Source: CAD feature listing. Evaluate the final solid. Frame: model axes, mm. Give positions to 0.01 mm unless a question says otherwise; leave off trailing zeros. Write each loop counter-clockwise with the first axis right and the second up, starting at its lowest first coordinate (ties: lowest second). Pieces come first, ordered by that corner, then holes. Notation, with made-up numbers: M 25.5,49.5 L 46.5,49.5 A35 ccw 46.5,86.5 Z; hole C -21.75,-6 d9. An arc over 180 degrees is marked long. Return JSON: item names as keys, results as strings.
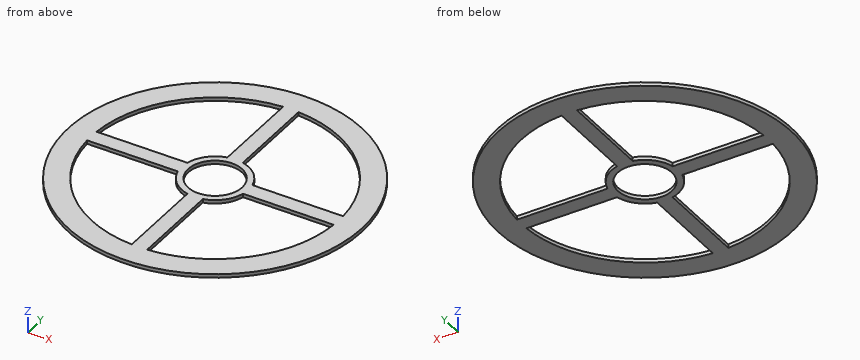
```python
from build123d import *

# Parameters (mm, degrees)
F0_R     = 28.5
F1_DEPTH = 0.7
F2_R     = 5.25
F3_DEPTH = 0.7
F5_DEPTH = 0.7


with BuildPart() as f1:
    # F0 (on Top) → F1 (new body)
    with BuildSketch(Plane.XY):
        Circle(F0_R)
    extrude(amount=F1_DEPTH)

    # F2 (on face) → F3 (cut, through all)
    with BuildSketch(Plane.XY.offset(0.7)):
        Circle(F2_R)
    extrude(amount=-F3_DEPTH, mode=Mode.SUBTRACT)

    # F4 (on face) → F5 (cut, through all)
    with BuildSketch(Plane.XY.offset(0.7)):
        with BuildLine():
            Line((-1.500154, 6.324555), (-1.500154, 23.953079))
            ThreePointArc((-1.500154, 23.953079), (-16.970717, 16.970563), (-23.953233, 1.5))
            Line((-23.953233, 1.5), (-6.324709, 1.5))
            ThreePointArc((-6.324709, 1.5), (-4.596348, 4.596194), (-1.500154, 6.324555))
        make_face()
        with BuildLine():
            Line((6.324401, 1.5), (23.952925, 1.5))
            ThreePointArc((23.952925, 1.5), (16.970409, 16.970563), (1.499846, 23.953079))
            Line((1.499846, 23.953079), (1.499846, 6.324555))
            ThreePointArc((1.499846, 6.324555), (4.59604, 4.596194), (6.324401, 1.5))
        make_face()
        with BuildLine():
            ThreePointArc((1.499846, -23.953079), (16.970409, -16.970563), (23.952925, -1.5))
            Line((23.952925, -1.5), (6.324401, -1.5))
            ThreePointArc((6.324401, -1.5), (4.59604, -4.596194), (1.499846, -6.324555))
            Line((1.499846, -6.324555), (1.499846, -23.953079))
        make_face()
        with BuildLine():
            ThreePointArc((-23.953233, -1.5), (-16.970717, -16.970563), (-1.500154, -23.953079))
            Line((-1.500154, -23.953079), (-1.500154, -6.324555))
            ThreePointArc((-1.500154, -6.324555), (-4.596348, -4.596194), (-6.324709, -1.5))
            Line((-6.324709, -1.5), (-23.953233, -1.5))
        make_face()
    extrude(amount=-F5_DEPTH, mode=Mode.SUBTRACT)


solid = f1.part
```
1) Line query: line 1 (Y direction, x = 0, z = 0.5); line 2 (X direction, y = -17, z = 0.25); line 3 (Y direction, x = -8, z = 0.3). Output: solid intervals per line, ascending. Write a range as [from, to].
Numbers:
{"line 1": "y = [-28.5, -5.25], [5.25, 28.5]", "line 2": "x = [-22.87, -16.94], [-1.5, 1.5], [16.94, 22.87]", "line 3": "y = [-27.35, -22.63], [-1.5, 1.5], [22.63, 27.35]"}
2) Cut plane C-C, the plane y = 10.5. Return the cut outline in (x, z).
Numbers:
{"outline": "M -26.5,0 L -21.58,0 L -21.58,0.7 L -26.5,0.7 Z; M -1.5,0 L 1.5,0 L 1.5,0.7 L -1.5,0.7 Z; M 21.58,0 L 26.5,0 L 26.5,0.7 L 21.58,0.7 Z"}
3) Cut plane A-A, the plane x = 0. Return the cut outline in (y, z).
Numbers:
{"outline": "M -28.5,0 L -5.25,0 L -5.25,0.7 L -28.5,0.7 Z; M 5.25,0 L 28.5,0 L 28.5,0.7 L 5.25,0.7 Z"}
4) Contact query for a flat-ended pin moving along its axis: pin 1 Ø10 at (x, y) = (10, -22) entering from -Z. Output: stop coordinate, or through.
Numbers:
{"pin 1": "stops at z = 0"}
5) Cut plane D-D, the plane x = 12. Return the cut outline in (y, z).
Numbers:
{"outline": "M -25.85,0 L -20.78,0 L -20.78,0.7 L -25.85,0.7 Z; M -1.5,0 L 1.5,0 L 1.5,0.7 L -1.5,0.7 Z; M 20.78,0 L 25.85,0 L 25.85,0.7 L 20.78,0.7 Z"}
